```python
from build123d import *

# Parameters (mm, degrees)
SKETCH1_W           = 36
SKETCH1_H           = 30
BOSS_EXTRUDE1_DEPTH = 3
SKETCH2_W           = 13.789302678
SKETCH2_H           = 8.180966888
BOSS_EXTRUDE2_DEPTH = 30
FILLET1_R           = 2
FILLET2_R           = 7
SKETCH3_R           = 4
CUT_EXTRUDE1_DEPTH  = 13
SKETCH1_4_R         = 2
CUT_EXTRUDE2_DEPTH  = 4


with BuildPart() as part:
    # Sketch1 → Boss-Extrude1 (new body)
    with BuildSketch(Plane(origin=(0, 0, 0), x_dir=(1, 0, 0), z_dir=(0, 1, 0))):
        Rectangle(SKETCH1_W, SKETCH1_H)
    extrude(amount=BOSS_EXTRUDE1_DEPTH)

    # Sketch2 → Boss-Extrude2 (add)
    with BuildSketch(Plane(origin=(0, 3, 0), x_dir=(1, 0, 0), z_dir=(0, 1, 0))):
        Rectangle(SKETCH2_W, SKETCH2_H)
    extrude(amount=BOSS_EXTRUDE2_DEPTH)

    # Fillet1
    fillet1_edges = [part.edges().sort_by_distance(p)[0] for p in [
        (-18, 1.5, 15),
        (18, 1.5, 15),
        (18, 1.5, -15),
        (-18, 1.5, -15),
    ]]
    fillet(fillet1_edges, radius=FILLET1_R)

    # Fillet2
    # the kernel refuses this fillet: 7 mm, written as the material it takes off along each edge
    with BuildSketch(Plane(origin=(6.894651339, 33, 21.590483444), x_dir=(0, -1, 0), z_dir=(0, 0, -1)), Plane(origin=(-6.894651339, 33, -21.590483444), x_dir=(0, -1, 0), z_dir=(0, 0, 1))) as fillet2_piece_1:
        with BuildLine():
            CenterArc((FILLET2_R, FILLET2_R), FILLET2_R, 180, 90)
            Line((0, FILLET2_R), (0, 0))
            Line((0, 0), (FILLET2_R, 0))
        make_face()
    extrude(amount=43.180966887, mode=Mode.SUBTRACT)

    # Sketch3 → Cut-Extrude1 (cut)
    with BuildSketch(Plane.XY.offset(4.090483444)):
        with Locations((0, 27)):
            Circle(SKETCH3_R)
    extrude(amount=-CUT_EXTRUDE1_DEPTH, mode=Mode.SUBTRACT)

    # Sketch1<4> → Cut-Extrude2 (cut)
    with BuildSketch(Plane(origin=(0, 0, 0), x_dir=(1, 0, 0), z_dir=(0, 1, 0))):
        with Locations(Location((-14.5, 12.083333333, 0), (0, 0, 90))):
            Circle(SKETCH1_4_R)
        with Locations(Location((14.5, 12.083333333, 0), (0, 0, 90))):
            Circle(SKETCH1_4_R)
        with Locations(Location((14.5, -12.083333333, 0), (0, 0, 90))):
            Circle(SKETCH1_4_R)
        with Locations(Location((-14.5, -12.083333333, 0), (0, 0, 90))):
            Circle(SKETCH1_4_R)
    extrude(amount=CUT_EXTRUDE2_DEPTH, mode=Mode.SUBTRACT)


solid = part.part
```
Could you check a few things on this model? Use its own coordinates, in mm. A direction names the side the tool comes from. Round coordinates to 2 decimals unless told otherwise and drop trailing zeros. Write each loop counter-clockwise with the first axis right and the second up, starting at its lowest first coordinate (ties: lowest second). Pieces come first, ordered by that corner, then holes. Notation, with made-up numbers: M -2,-29.75 L 44,-29.75 A6 cw 44,-23.75 Z; hole C -16,74.5 d8. An arc over 180 degrees is marked long. Answer in a Markdown table with one row per item. Add a question column.
Q1. If we mould it in two halves opening along X, with no side actions, what happens to faces 1 (the cylindrical face through (-16.186, 1.479, 11.008)), 2 (the cylindrical face through (-17.43, 1.52, -14.4)), 3 (the flat face through (18, 1, 0)), 4 (the flat face through (0, 0, 0))? For each: +X half, -X half, draft (parallel to the pull), parting line (faces both ways), or undercut.
Q2. Imagine slicing it at B-B (y = 29). Please give me the cut outline in (x, z).
Q3. Imagine slicing it at A-A (x = 14.5). Please give me the cut outline in (y, z).
Q4. Will these pins go through, and if not, where does the flat tip stop? pin 1 Ø6.5 at (y, z) = (16, -2) entering from -X; pin 2 Ø10 at (x, y) = (11, 22) entering from -Z; pin 3 Ø6 at (y, z) = (17.5, -9.5) entering from -X; pin 4 Ø6 at (x, y) = (-9, 26) entering from +Z.
Q5. Imagine slicing it at D-D (x = -2.5). Please give me the cut outline in (y, z).
Q6. Imagine slicing it at C-C (x = 6). Please give me the cut outline in (y, z), then the cut area to 3 significant figures.
Q7. If I drill on line 1 (Z direction, x = 14.5, y = 1.55); line 2 (Z direction, x = -14, y = 2); line 3 (X direction, y = 16, z = 0.5), over which ranges is the centre line in solid material (lowest first)? Write a range as from..to.
Q8. On a 3-axis mill with a long thin cutter (end or side, diameter ignored), from which of +Z, -Z, +X, -X, +Y, -Y can I reach the whole of each face in a straight line? I mean faces 5 (the flat face through (-6.895, 14, 0)), 6 (the flat face through (0, 14, -4.09)), 7 (the flat face through (0, 14, 4.09)). Say none if no direction works.
Values:
| question | item | result |
|---|---|---|
| 1 | face 1 | undercut |
| 1 | face 2 | -X half |
| 1 | face 3 | +X half |
| 1 | face 4 | draft |
| 2 | outline | M -6.22,-4.09 L -3.46,-4.09 L -3.46,4.09 L -6.22,4.09 Z; M 3.46,-4.09 L 6.22,-4.09 L 6.22,4.09 L 3.46,4.09 Z |
| 3 | outline | M 0,-15 L 3,-15 L 3,-14.08 L 0,-14.08 Z; M 0,-10.08 L 3,-10.08 L 3,10.08 L 0,10.08 Z; M 0,14.08 L 3,14.08 L 3,15 L 0,15 Z |
| 4 | pin 1 | x = -6.89 |
| 4 | pin 2 | z = -4.09 |
| 4 | pin 3 | through |
| 4 | pin 4 | z = 4.09 |
| 5 | outline | M 0,-15 L 3,-15 L 3,-4.09 L 23.88,-4.09 L 23.88,4.09 L 3,4.09 L 3,15 L 0,15 Z; M 30.12,-4.09 L 32.5,-4.09 L 32.5,4.09 L 30.12,4.09 Z |
| 6 | outline | M 0,-15 L 3,-15 L 3,-4.09 L 29.42,-4.09 L 29.42,4.09 L 3,4.09 L 3,15 L 0,15 Z |
| 6 | area | 306 mm^2 |
| 7 | line 1 | -15..-14.08, -10.08..10.08, 14.08..15 |
| 7 | line 2 | -15..-14.02, -10.15..10.15, 14.02..15 |
| 7 | line 3 | -6.89..6.89 |
| 8 | face 5 | +Z, -Z, -X, +Y |
| 8 | face 6 | -Z, +X, -X, +Y |
| 8 | face 7 | +Z, +X, -X, +Y |
